Read the model definition and answer for the solid it produces. Units are mm, in the model's axes. Face numbers are marked on the shaded views. A direction names the side the tool comes from. Give positions to 0.01 mm unless a question says otherwise; leave off trailing zeros. Order: outer loops, then holes, each group sorted by start corner. A loop starts at its lowest first (then second) coordinate and runs counter-clockwise, first axis right, second up. Notation, with made-up numbers: (44.5, -20) - (69.5, -20) arc R25 cw to (69.5, 4) - close; hole circle Ø1 at (10.5, -30.5). An arc over 180 degrees is marked (long way). One line per item, written item: value. Start each with the question number.
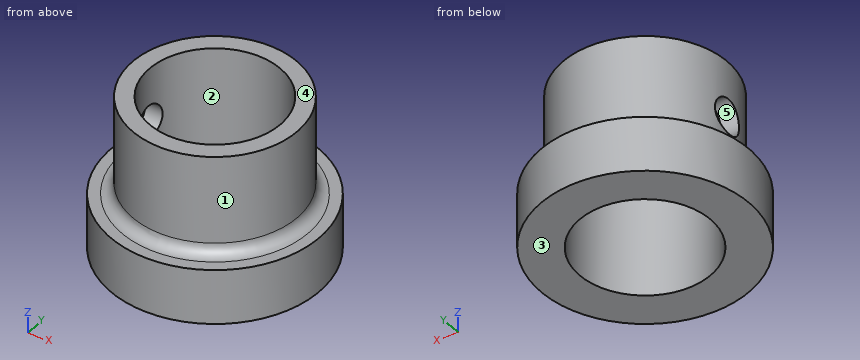
```python
from build123d import *

# Parameters (mm, degrees)
SKETCH2_R           = 7.5
SKETCH2_R_2         = 5.975
BOSS_EXTRUDE1_DEPTH = 9
SKETCH3_R           = 9.5
BOSS_EXTRUDE2_DEPTH = 5
CUT_EXTRUDE1_START  = -5
SKETCH4_R           = 5.975
CUT_EXTRUDE1_DEPTH  = 5
SKETCH5_R           = 1.6
CUT_EXTRUDE2_DEPTH  = 12
FILLET1_R           = 1


with BuildPart() as part:
    # Sketch2 → Boss-Extrude1 (new body)
    with BuildSketch(Plane.XY):
        Circle(SKETCH2_R)
        Circle(SKETCH2_R_2, mode=Mode.SUBTRACT)
    extrude(amount=BOSS_EXTRUDE1_DEPTH)

    # Sketch3 → Boss-Extrude2 (add)
    with BuildSketch(Plane(origin=(0, 0, 0), x_dir=(-1, 0, 0), z_dir=(0, 0, -1))):
        Circle(SKETCH3_R)
    extrude(amount=BOSS_EXTRUDE2_DEPTH)

    # Sketch4 → Cut-Extrude1 (cut)
    with BuildSketch(Plane.XY.offset(CUT_EXTRUDE1_START)):
        Circle(SKETCH4_R)
    extrude(amount=CUT_EXTRUDE1_DEPTH, mode=Mode.SUBTRACT)

    # Sketch5 → Cut-Extrude2 (cut)
    with BuildSketch(Plane.ZY.offset(7.5)):
        with Locations((4, 0)):
            Circle(SKETCH5_R)
    extrude(amount=-CUT_EXTRUDE2_DEPTH, mode=Mode.SUBTRACT)

    # Fillet1
    fillet1_edges = [part.edges().sort_by_distance(p)[0] for p in [
        (-7.5, 0, 0),
    ]]
    fillet(fillet1_edges, radius=FILLET1_R)


solid = part.part
```
1) Section A-A on x = 0 is taken. Write down the section's boundary in (y, z) (3 decimals), plus the area to 3 significant figures.
2) Section D-D on z = -3.75 is taken. Write down the section's boundary in (x, y) (3 decimals), plus the area to 3 significant figures.
3) For the marked faces 4 and 5, determine the directions among +Z, -Z, +X, -X, +Y, -Y from which every point of the face is accessible in a straight line to the end or side of a thin tool.
4) Find the intervals of material crossed by probe 1 along Y at (x, z) = (-6.5, 4); probe 2 along X at (y, z) = (-5.5, -1.75); probe 3 along X at (y, z) = (3.75, 6.25), in increasing order. Write a range as from..to.
5) Section C-C on z = 6 is taken. Write down the section's boundary in (x, y) (3 decimals), plus the area to 3 significant figures.
6) Each of these flat-tipped pins is pushed along its axis until it touches: pin 1 (5 mm diameter, centred on x = -3, z = 0.5, fed in from +Y); pin 2 (1 mm diameter, centred on y = -7, z = -3, fed in from -X); pin 3 (1.5 mm diameter, centred on x = -2, z = 5.5, fed in from +Y). Where does it stop, or does it pass through?
7) Section B-B on y = 0 is taken. Write down the section's boundary in (x, z) (3 decimals).
8) The mould has two halves that part along Y. Classify the marked faces 1, 2 and 3: +Y half, -Y half, draft (parallel to the pull), parting line (faces both ways), or undercut.
Solved:
1. outline: (-9.5, -5) - (-5.975, -5) - (-5.975, 9) - (-7.5, 9) - (-7.5, 1) arc R1 cw to (-8.5, 0) - (-9.5, 0) - close; (5.975, -5) - (9.5, -5) - (9.5, 0) - (8.5, 0) arc R1 cw to (7.5, 1) - (7.5, 9) - (5.975, 9) - close
1. area: 63.1 mm2
2. outline: circle Ø19 at (0, 0); hole circle Ø11.95 at (0, 0)
2. area: 171 mm2
3. face 4: +Z, +X, -X, +Y, -Y
3. face 5: -X
4. probe 1: y = -3.74..-1.6, 1.6..3.74
4. probe 2: x = -7.75..-2.33, 2.33..7.75
4. probe 3: x = -6.5..-4.65, 4.65..6.5
5. outline: circle Ø15 at (0, 0); hole circle Ø11.95 at (0, 0)
5. area: 64.6 mm2
6. pin 1: stops at y = 9.48
6. pin 2: stops at x = -6.93
6. pin 3: stops at y = 7.4
7. outline: (-9.5, -5) - (-5.975, -5) - (-5.975, 2.4) - (-7.5, 2.4) - (-7.5, 1) arc R1 cw to (-8.5, 0) - (-9.5, 0) - close; (-7.5, 5.6) - (-5.975, 5.6) - (-5.975, 9) - (-7.5, 9) - close; (5.975, -5) - (9.5, -5) - (9.5, 0) - (8.5, 0) arc R1 cw to (7.5, 1) - (7.5, 9) - (5.975, 9) - close
8. face 1: parting line
8. face 2: undercut
8. face 3: draft
